```python
from build123d import *

# Parameters (mm, degrees)
PAD_DEPTH = 25


with BuildPart() as part:
    # Sketch → Pad (new body)
    with BuildSketch(Plane.XY):
        with BuildLine():
            ThreePointArc((64, 24), (50.400723, 45.68526), (24.965644, 42.813397))
            ThreePointArc((24.965644, 42.813397), (24.179475, 35.786169), (31.206703, 35))
            ThreePointArc((39.96481, 10), (53.210772, 28.674471), (31.206703, 35))
            Line((39.96481, 10), (24.965644, 10))
            Line((24.965644, 10), (0, 0))
            Line((0, 0), (64, 0))
            Line((64, 0), (64, 24))
        make_face()
    extrude(amount=PAD_DEPTH)


solid = part.part
```
Can you work these out from the model? Positions are in its coordinate system, mm. A direction names the side the tool comes from. Coordinates: 2 decimals unless noted, no trailing zeros. Order: outer loops, then holes, each group sorted by start corner. A loop starts at its lowest first (then second) coordinate and runs counter-clockwise, first axis right, second up. Notation, with made-up numbers: (44.5, 80.25) - (59.5, 80.25) arc R26 cw to (59.5, 118.25) - close; hole circle Ø7 at (65.25, 86). An arc over 180 degrees is marked (long way). Answer in a Markdown table with one row per item.
1. Suppose I cut it at A-A (x = 51.5). Please give me the cut outline in (y, z).
Reply:
| item | result |
|---|---|
| outline | (0, 0) - (16.04, 0) - (16.04, 25) - (0, 25) - close; (32.03, 0) - (45.12, 0) - (45.12, 25) - (32.03, 25) - close |
2. For pin 1 (3 mm diameter, centred on y = 5, z = 21, fed in from -X); pin 2 (6 mm diameter, centred on x = 25.5, z = 21, fed in from +Y); pin 3 (5 mm diameter, centred on x = 18, z = 3, fed in from +Y), each with a flat end and sliding along its axis, tell me the tip position at first contact or that it passes through.
Reply:
| item | result |
|---|---|
| pin 1 | stops at x = 8.74 |
| pin 2 | stops at y = 45.16 |
| pin 3 | stops at y = 8.21 |
3. If I drill on line 1 along Y through (x, z) = (35.5, 3); line 2 along Y through (x, z) = (23.5, 7); line 3 along Y through (x, z) = (61.5, 4.5), over which ranges is the centre line in solid material (lowest first)?
Reply:
| item | result |
|---|---|
| line 1 | y = 0 to 10, 37.34 to 47.65 |
| line 2 | y = 0 to 9.41, 36.91 to 40.9 |
| line 3 | y = 0 to 34.71 |
4. Suppose I cut it at C-C (y = 37). Please give me the cut outline in (x, z), and give its area (3 significant figures).
Reply:
| item | result |
|---|---|
| outline | (23.46, 0) - (34.59, 0) - (34.59, 25) - (23.46, 25) - close; (45.34, 0) - (60.2, 0) - (60.2, 25) - (45.34, 25) - close |
| area | 650 mm^2 |
5. For faces 1 (the flat face through (53, 14, 25)), 2 (the flat face through (33, 10, 12)), which set-ups out of +Z, -Z, +X, -X, +Y, -Y let a thin tool reach every point of the face, with its end or its side?
Reply:
| item | result |
|---|---|
| face 1 | +Z, +X, -X, +Y, -Y |
| face 2 | +Z, -Z, -X |
6. If we mould it in two halves opening along X, with no side actions, what happens to faces 3 (the cylindrical face through (53.33, 28.32, 12.32)), 4 (the flat face through (53, 14, 0)), 5 (the cylindrical face through (24.112, 35.873, 12.325)), 6 (the flat face through (12.66, 5.07, 12.32))? For each: pulls with the +X half, pulls with the -X half, needs draft (parallel to the pull), parting line crosses it, or undercut.
Reply:
| item | result |
|---|---|
| face 3 | undercut |
| face 4 | needs draft |
| face 5 | undercut |
| face 6 | pulls with the -X half |
7. Suppose I cut it at D-D (x = 15). Please give me the cut outline in (y, z), and give its area (3 significant figures).
Reply:
| item | result |
|---|---|
| outline | (0, 0) - (6.01, 0) - (6.01, 25) - (0, 25) - close |
| area | 150 mm^2 |
8. Suppose I cut it at B-B (z = 17). Please give me the cut outline in (x, y), and give its area (3 significant figures).
Reply:
| item | result |
|---|---|
| outline | (0, 0) - (64, 0) - (64, 24) arc R24.03 ccw to (24.97, 42.81) arc R5 ccw to (31.21, 35) arc R14.03 cw (long way) to (39.96, 10) - (24.97, 10) - close |
| area | 1,160 mm^2 |
